from build123d import *

# Parameters (mm, degrees)
SKETCH1_W           = 119.6
SKETCH1_H           = 24
BOSS_EXTRUDE1_DEPTH = 9.7
SKETCH3_W           = 9.4
SKETCH3_H           = 13.2
BOSS_EXTRUDE2_DEPTH = 8
SKETCH4_R           = 0.95
CUT_EXTRUDE1_DEPTH  = 71.971050436


with BuildPart() as part:
    # Sketch1 → Boss-Extrude1 (new body)
    with BuildSketch(Plane.YZ):
        Rectangle(SKETCH1_W, SKETCH1_H)
    extrude(amount=BOSS_EXTRUDE1_DEPTH)

    # Sketch3 → Boss-Extrude2 (add)
    with BuildSketch(Plane(origin=(0, 59.8, 0), x_dir=(-1, 0, 0), z_dir=(0, 1, 0))):
        with Locations((-4.7, 0)):
            Rectangle(SKETCH3_W, SKETCH3_H)
    extrude(amount=BOSS_EXTRUDE2_DEPTH)

    # Sketch4 → Cut-Extrude1 (cut, through all)
    with BuildSketch(Plane.XY.offset(6.6)):
        with BuildLine():
            Line((0, 67.8), (0, 64.1))
            ThreePointArc((0, 64.1), (4.7, 67.5), (9.4, 64.1))
            Line((9.4, 64.1), (9.4, 67.8))
            Line((9.4, 67.8), (0, 67.8))
        make_face()
        with Locations((4, 64.1)):
            Circle(SKETCH4_R)
    extrude(amount=-CUT_EXTRUDE1_DEPTH, mode=Mode.SUBTRACT)


solid = part.part
Can you work these out from the model? Positions are in its coordinate system, mm. A direction names the side the tool comes from. Coordinates: 2 decimals unless noted, no trailing zeros. Order: outer loops, then holes, each group sorted by start corner. A loop starts at its lowest first (then second) coordinate and runs counter-clockwise, first axis right, second up. Notation, with made-up numbers: (12, 35.5) -> (56, 35.5) arc R34 cw to (56, 65.5) -> close; hole circle Ø4 at (29, 32.5). An arc over 180 degrees is marked (long way). Use one line per item in the form item = value.
Q1. Will these pins go through, and if not, where does the flat tip stop? P1, Ø4.5, axis at y = 62.5, z = -0.5, coming from the +X side; P2, Ø2.5, axis at x = 4, y = 64.1, coming from the -Z side; P3, Ø2.5, axis at x = 4.5, y = 62.5, coming from the +Z side.
From the geometry:
P1 = 9.4
P2 = -6.6
P3 = 6.6
Q2. I need wall thicknesses on L1, parallel to X at y = 64.1, z = -1; L2, parallel to Y at x = 7.5, z = -8; L3, parallel to Y at x = 4, z = 1. Which ranges of each line are inside material? Lowest first, please.
From the geometry:
L1 = 0 to 3.05, 4.95 to 9.4
L2 = -59.8 to 59.8
L3 = -59.8 to 63.15, 65.05 to 67.45
Q3. Imagine slicing it at A-A, the plane x = 6.5. List the corners of the cut face in (y, z) for me, then the cut area to 3 significant figures.
From the geometry:
outline = (-59.8, -12) -> (59.8, -12) -> (59.8, -6.6) -> (67.16, -6.6) -> (67.16, 6.6) -> (59.8, 6.6) -> (59.8, 12) -> (-59.8, 12) -> close
area = 2,970 mm²
Q4. Which directions (+Z, -Z, +X, -X, +Y, -Y) give clear straight access to the entire face, cutting with the end or side of a thin tool? Please do faces 1 (the face through (5, 63, -6.6)), 2 (the face through (5, 63, 6.6)), 3 (the face through (9.4, 62, 0)).
From the geometry:
face_1 = -Z, +X, -X, +Y
face_2 = +Z, +X, -X, +Y
face_3 = +Z, -Z, +X, +Y
Q5. Imagine slicing it at B-B, the plane z = -9.5. List the corners of the cut face in (x, y) for me.
From the geometry:
outline = (0, -59.8) -> (9.7, -59.8) -> (9.7, 59.8) -> (0, 59.8) -> close
